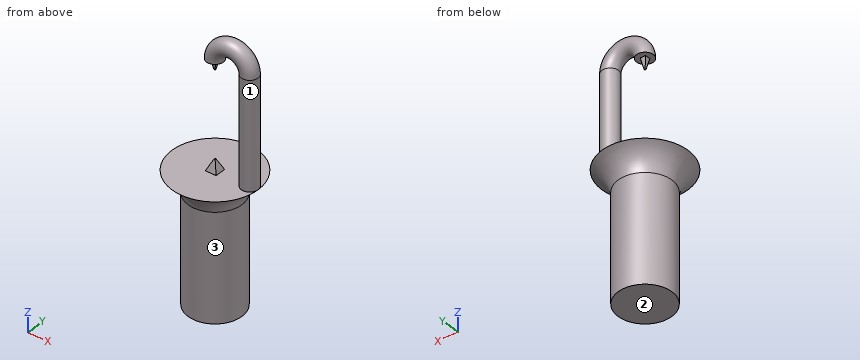
```python
from build123d import *

# Parameters (mm, degrees)
F0_W     = 31.75
F0_H     = 127
F2_R     = 9.8908810496
F3_DEPTH = 127
F4_W     = 12.7
F4_H     = 12.7
F6_W     = 1.27
F6_H     = 1.27
F8_R     = 9.8775603936
F9_ANGLE = 180
F12_W    = 6.35
F12_H    = 6.35
F11_W    = 1.27
F11_H    = 1.27


with BuildPart() as f1:
    # F0 (on Front) → F1 (revolve)
    with BuildSketch(Plane.XZ):
        with BuildLine():
            Line((0, 152.4), (0, 127))
            Line((0, 127), (31.75, 127))
            ThreePointArc((31.75, 127), (38.1902000249, 142.0135999813), (50.8, 152.4))
            Line((50.8, 152.4), (0, 152.4))
        make_face()
        with Locations((15.875, 63.5)):
            Rectangle(F0_W, F0_H)
    revolve(axis=Axis((0, 0, 63.5), (0, 0, 1)))

    # F2 (on face) → F3 (join)
    with BuildSketch(Plane.XY.offset(152.4)):
        with Locations((40.9091189504, 0)):
            Circle(F2_R)
    extrude(amount=F3_DEPTH)

    # F4 (on face) → F7 section 0
    with BuildSketch(Plane.XY.offset(152.4)):
        Rectangle(F4_W, F4_H)
    # F6 (on offset) → F7 section 1
    with BuildSketch(Plane.XY.offset(165.1)):
        Rectangle(F6_W, F6_H)
    loft()

    # F8 (on face) → F9 (revolve)
    with BuildSketch(Plane.XY.offset(279.4)):
        with Locations((40.9091189504, 0)):
            Circle(F8_R)
    revolve(axis=Axis((20.4545594752, 1.762766391, 279.4), (0, -1, 0)), revolution_arc=F9_ANGLE)

    # F12 (on face) → F13 section 0
    with BuildSketch(Plane(origin=(0, 0, 279.4), x_dir=(1, 0, 0), z_dir=(0, 0, -1))):
        Rectangle(F12_W, F12_H)
    # F11 (on offset) → F13 section 1
    with BuildSketch(Plane(origin=(0, 0, 266.7), x_dir=(1, 0, 0), z_dir=(0, 0, -1))):
        Rectangle(F11_W, F11_H)
    loft()


solid = f1.part
```
Could you check a few things on this model? Use its own coordinates, in mm. Face numbers are marked on the shaded views. Coordinates: 2 decimals unless noted, no trailing zeros. Order: outer loops, then holes, each group sorted by start corner. A loop starts at its lowest first (then second) coordinate and runs counter-clockwise, first axis right, second up. Notation, with made-up numbers: M -24.5,31.5 L 5.5,31.5 A15 cw 5.5,44.5 Z; hole C 61.25,35 d9. An arc over 180 degrees is marked long. Use one line per item in the form item = value. Start each with the question number.
1. For pin 1 (10 mm diameter, centred on x = 43.5, y = 3, fed in from +Z); pin 2 (12 mm diameter, centred on x = 26.5, y = 0, fed in from -Z); pin 3 (12 mm diameter, centred on y = 0.5, z = 248, fed in from -X); pin 4 (3 mm diameter, centred on x = -21, z = 101.5, fed in from -Y), each with a flat end and sliding along its axis, tell me the tip position at first contact or that it passes through.
2. Please list where these lines run through material, in increasing order: line 1 (Z direction, x = 13, y = -15.5); line 2 (Z direction, x = 4, y = -7); line 3 (X direction, y = 6, z = 16).
3. We'd pull the mould along Z, two halves only. Please class the marked faces 1, 2 and 3: +Z half, -Z half, draft (parallel to the pull), parting line (faces both ways), or undercut.
4. Suppose I cut it at B-B on z = 81. Write out the boundary of the cut face in (x, y), then the cut area to 3 significant figures.
5. Suppose I cut it at A-A on z = 171. Write out the boundary of the cut face in (x, y).
Geometry says:
q1.pin_1 = 303.47
q1.pin_2 = 0
q1.pin_3 = 31.02
q1.pin_4 = -25.06
q2.line_1 = 0 to 152.4
q2.line_2 = 0 to 152.4, 279.4 to 301.34
q2.line_3 = -31.18 to 31.18
q3.face_1 = undercut
q3.face_2 = -Z half
q3.face_3 = draft
q4.outline = C 0,0 d63.5
q4.area = 3,170 mm^2
q5.outline = C 40.91,0 d19.78
